from build123d import *

# Parameters (mm, degrees)
SKETCH1_W                        = 190
SKETCH1_H                        = 120
BOSS_EXTRUDE1_DEPTH              = 170
SKETCH2_W                        = 50
SKETCH2_H                        = 75
CUT_EXTRUDE1_DEPTH               = 190
CUT_EXTRUDE2_DEPTH               = 15
CUT_EXTRUDE3_DEPTH               = 15
CUT_EXTRUDE4_DEPTH               = 15
M10X1_0_TAPPED_HOLE1_D           = 9
M10X1_0_TAPPED_HOLE1_DEPTH       = 23
M10X1_0_TAPPED_HOLE1_CBORE_D     = 10
M10X1_0_TAPPED_HOLE1_CBORE_DEPTH = 20
M10X1_0_TAPPED_HOLE1_TIP         = 2.703872786
M10X1_0_TAPPED_HOLE2_D           = 9
M10X1_0_TAPPED_HOLE2_DEPTH       = 23
M10X1_0_TAPPED_HOLE2_CBORE_D     = 10
M10X1_0_TAPPED_HOLE2_CBORE_DEPTH = 20
M10X1_0_TAPPED_HOLE2_TIP         = 2.703872786
M10X1_0_TAPPED_HOLE3_D           = 9
M10X1_0_TAPPED_HOLE3_DEPTH       = 23
M10X1_0_TAPPED_HOLE3_CBORE_D     = 10
M10X1_0_TAPPED_HOLE3_CBORE_DEPTH = 20
M10X1_0_TAPPED_HOLE3_TIP         = 2.703872786
M10X1_0_TAPPED_HOLE4_D           = 9
M10X1_0_TAPPED_HOLE4_DEPTH       = 23
M10X1_0_TAPPED_HOLE4_CBORE_D     = 10
M10X1_0_TAPPED_HOLE4_CBORE_DEPTH = 20
M10X1_0_TAPPED_HOLE4_TIP         = 2.703872786
M10X1_0_TAPPED_HOLE5_D           = 9
M10X1_0_TAPPED_HOLE5_DEPTH       = 23
M10X1_0_TAPPED_HOLE5_CBORE_D     = 10
M10X1_0_TAPPED_HOLE5_CBORE_DEPTH = 20
M10X1_0_TAPPED_HOLE5_TIP         = 2.703872786


with BuildPart() as part:
    # Sketch1 → Boss-Extrude1 (new body)
    with BuildSketch(Plane(origin=(0, 0, 0), x_dir=(1, 0, 0), z_dir=(0, 1, 0))):
        Rectangle(SKETCH1_W, SKETCH1_H)
    extrude(amount=BOSS_EXTRUDE1_DEPTH)

    # Sketch2 → Cut-Extrude1 (cut)
    with BuildSketch(Plane(origin=(95, 0, 0), x_dir=(0, 0, -1), z_dir=(1, 0, 0))):
        with Locations((-25, 122.5)):
            Rectangle(SKETCH2_W, SKETCH2_H)
        with Locations((25, 122.5)):
            Rectangle(SKETCH2_W, SKETCH2_H)
        with Locations((25, 47.5)):
            Rectangle(SKETCH2_W, SKETCH2_H)
        with Locations((-25, 47.5)):
            Rectangle(SKETCH2_W, SKETCH2_H)
    extrude(amount=-CUT_EXTRUDE1_DEPTH, mode=Mode.SUBTRACT)

    # Sketch3 → Cut-Extrude2 (cut)
    with BuildSketch(Plane.XY.offset(60)):
        with BuildLine():
            Line((-25, 80), (25, 80))
            ThreePointArc((25, 80), (32.071067812, 82.928932188), (35, 90))
            Line((35, 90), (35, 130))
            ThreePointArc((35, 130), (32.071067812, 137.071067812), (25, 140))
            Line((25, 140), (-25, 140))
            ThreePointArc((-25, 140), (-32.071067812, 137.071067812), (-35, 130))
            Line((-35, 130), (-35, 90))
            ThreePointArc((-35, 90), (-32.071067812, 82.928932188), (-25, 80))
        make_face()
    extrude(amount=-CUT_EXTRUDE2_DEPTH, mode=Mode.SUBTRACT)

    # Sketch4 → Cut-Extrude3 (cut)
    with BuildSketch(Plane(origin=(0, 0, -60), x_dir=(-1, 0, 0), z_dir=(0, 0, -1))):
        with BuildLine():
            Line((-25, 80), (25, 80))
            ThreePointArc((25, 80), (32.071067812, 82.928932188), (35, 90))
            Line((35, 90), (35, 130))
            ThreePointArc((35, 130), (32.071067812, 137.071067812), (25, 140))
            Line((25, 140), (-25, 140))
            ThreePointArc((-25, 140), (-32.071067812, 137.071067812), (-35, 130))
            Line((-35, 130), (-35, 90))
            ThreePointArc((-35, 90), (-32.071067812, 82.928932188), (-25, 80))
        make_face()
    extrude(amount=-CUT_EXTRUDE3_DEPTH, mode=Mode.SUBTRACT)

    # Sketch5 → Cut-Extrude4 (cut)
    with BuildSketch(Plane(origin=(0, 170, 0), x_dir=(1, 0, 0), z_dir=(0, 1, 0))):
        with BuildLine():
            Line((-25, -30), (25, -30))
            ThreePointArc((25, -30), (32.071067812, -27.071067812), (35, -20))
            Line((35, -20), (35, 20))
            ThreePointArc((35, 20), (32.071067812, 27.071067812), (25, 30))
            Line((25, 30), (-25, 30))
            ThreePointArc((-25, 30), (-32.071067812, 27.071067812), (-35, 20))
            Line((-35, 20), (-35, -20))
            ThreePointArc((-35, -20), (-32.071067812, -27.071067812), (-25, -30))
        make_face()
    extrude(amount=-CUT_EXTRUDE4_DEPTH, mode=Mode.SUBTRACT)

    # M10x1.0 Tapped Hole1
    with Locations(Plane(origin=(65, 110, -70), x_dir=(-1, 0, 0), z_dir=(0, 0, -1))):
        with Locations((0, 0), (130, 0), (62.5, -65)):
            CounterBoreHole(M10X1_0_TAPPED_HOLE1_D / 2, M10X1_0_TAPPED_HOLE1_CBORE_D / 2, M10X1_0_TAPPED_HOLE1_CBORE_DEPTH, depth=M10X1_0_TAPPED_HOLE1_DEPTH)
            with Locations((0, 0, -(M10X1_0_TAPPED_HOLE1_DEPTH + M10X1_0_TAPPED_HOLE1_TIP / 2))):  # 118° drill point
                Cone(0, M10X1_0_TAPPED_HOLE1_D / 2, M10X1_0_TAPPED_HOLE1_TIP, mode=Mode.SUBTRACT)

    # M10x1.0 Tapped Hole2
    with Locations(Plane(origin=(-65, 170, 0), x_dir=(0, 0, 1), z_dir=(0, 1, 0))):
        with Locations((0, 0), (0, 130)):
            CounterBoreHole(M10X1_0_TAPPED_HOLE2_D / 2, M10X1_0_TAPPED_HOLE2_CBORE_D / 2, M10X1_0_TAPPED_HOLE2_CBORE_DEPTH, depth=M10X1_0_TAPPED_HOLE2_DEPTH)
            with Locations((0, 0, -(M10X1_0_TAPPED_HOLE2_DEPTH + M10X1_0_TAPPED_HOLE2_TIP / 2))):  # 118° drill point
                Cone(0, M10X1_0_TAPPED_HOLE2_D / 2, M10X1_0_TAPPED_HOLE2_TIP, mode=Mode.SUBTRACT)

    # M10x1.0 Tapped Hole3
    with Locations(Plane(origin=(-65, 110, 60), x_dir=(1, 0, 0), z_dir=(0, 0, 1))):
        with Locations((0, 0), (130, 0), (67.5, -65), (67.5, 38)):
            CounterBoreHole(M10X1_0_TAPPED_HOLE3_D / 2, M10X1_0_TAPPED_HOLE3_CBORE_D / 2, M10X1_0_TAPPED_HOLE3_CBORE_DEPTH, depth=M10X1_0_TAPPED_HOLE3_DEPTH)
            with Locations((0, 0, -(M10X1_0_TAPPED_HOLE3_DEPTH + M10X1_0_TAPPED_HOLE3_TIP / 2))):  # 118° drill point
                Cone(0, M10X1_0_TAPPED_HOLE3_D / 2, M10X1_0_TAPPED_HOLE3_TIP, mode=Mode.SUBTRACT)

    # M10x1.0 Tapped Hole4
    with Locations(Plane(origin=(65, 0, 0), x_dir=(0, 0, -1), z_dir=(0, -1, 0))):
        with Locations((0, 0), (0, -130)):
            CounterBoreHole(M10X1_0_TAPPED_HOLE4_D / 2, M10X1_0_TAPPED_HOLE4_CBORE_D / 2, M10X1_0_TAPPED_HOLE4_CBORE_DEPTH, depth=M10X1_0_TAPPED_HOLE4_DEPTH)
            with Locations((0, 0, -(M10X1_0_TAPPED_HOLE4_DEPTH + M10X1_0_TAPPED_HOLE4_TIP / 2))):  # 118° drill point
                Cone(0, M10X1_0_TAPPED_HOLE4_D / 2, M10X1_0_TAPPED_HOLE4_TIP, mode=Mode.SUBTRACT)

    # M10x1.0 Tapped Hole5
    with Locations(Plane(origin=(-30, 20, 60), x_dir=(1, 0, 0), z_dir=(0, 0, 1))):
        with Locations((0, 0), (60, 0)):
            CounterBoreHole(M10X1_0_TAPPED_HOLE5_D / 2, M10X1_0_TAPPED_HOLE5_CBORE_D / 2, M10X1_0_TAPPED_HOLE5_CBORE_DEPTH, depth=M10X1_0_TAPPED_HOLE5_DEPTH)
            with Locations((0, 0, -(M10X1_0_TAPPED_HOLE5_DEPTH + M10X1_0_TAPPED_HOLE5_TIP / 2))):  # 118° drill point
                Cone(0, M10X1_0_TAPPED_HOLE5_D / 2, M10X1_0_TAPPED_HOLE5_TIP, mode=Mode.SUBTRACT)


solid = part.part
Work out the finished part from the listing and answer in its coordinate system (mm). A direction names the side the tool comes from. Coordinates: 2 decimals unless noted, no trailing zeros. Write each loop counter-clockwise with the first axis right and the second up, starting at its lowest first coordinate (ties: lowest second). Pieces come first, ordered by that corner, then holes.
1. For a pull along Z with two mould halves and no side action, classify faces 1 (the cylindrical face through (-63.92, 105.12, -55.07)), 2 (the cylindrical face through (-32.15, 165.07, 26.99)) as +Z half, -Z half, draft (parallel to the pull), parting line (faces both ways), or undercut.
Results list:
face 1: draft
face 2: undercut
2. Consider line 1 along Y through (x, z) = (2.5, -55); line 2 along X through (y, z) = (163, 0); line 3 along Z through (x, y) = (-57, 111.5). Determine where each line is inside the solid, lowest interval first.
Results list:
line 1: y = 0 to 40, 50 to 80, 140 to 170
line 2: x = -95 to -70, -60 to -35, 35 to 60, 70 to 95
line 3: z = -60 to -50, 50 to 60
3. The part is cut by section A-A, the plane x = 2.5. State how many separate pieces and enclosed holes the cut face has, and give its area (3 significant figures).
Results list:
separate pieces: 6
enclosed holes: 0
area: 3,300 mm2
4. The part is cut by section B-B, the plane y = 45. Write down the section's boundary in (x, z), and give its area (3 significant figures).
Results list:
outline: (-95, -60) - (-2.5, -60) - (-2.5, -50) - (-95, -50) - close; (-95, 50) - (-2.5, 50) - (-2.5, 60) - (-95, 60) - close; (7.5, -60) - (95, -60) - (95, -50) - (7.5, -50) - close; (7.5, 50) - (95, 50) - (95, 60) - (7.5, 60) - close
area: 3,600 mm2
5. The part is cut by section D-D, the plane y = 148. Write down the section's boundary in (x, z), and give its area (3 significant figures).
Results list:
outline: (-95, -60) - (95, -60) - (95, -50) - (-95, -50) - close; (-95, 50) - (-2.5, 50) - (-2.5, 60) - (-95, 60) - close; (7.5, 50) - (95, 50) - (95, 60) - (7.5, 60) - close
area: 3,700 mm2
6. For faces 3 (the cylindrical face through (32.15, 165.07, -26.99)), 4 (the cylindrical face through (26, 17, 55)), 5 (the flat face through (1, 160, -34)), 6 (the cylindrical face through (32.15, 83.01, -55.07)), determine the directions among +Z, -Z, +X, -X, +Y, -Y from which every point of the face is accessible in a straight line to the end or side of a thin tool.
Results list:
face 3: +Y
face 4: +Z
face 5: +X, -X
face 6: +Z, -Z
7. The part is cut by section C-C, the plane z = 14.5. Write down the section's boundary in (x, y).
Results list:
outline: (-95, 0) - (95, 0) - (95, 10) - (-95, 10) - close; (-95, 160) - (-35, 160) - (-35, 170) - (-95, 170) - close; (35, 160) - (95, 160) - (95, 170) - (35, 170) - close
8. A flat-ended cylindrical pin translates along its axis: pin 1 (8 mm diameter, centred on x = -65, y = 110, fed in from +Z). Find the tip coordinate at first contact, or state that the pin passes through.
Results list:
pin 1: passes through
